Geometry: final body of the model. Coordinates: model frame, mm. Coordinates: 2 decimals unless noted, no trailing zeros. Write each loop counter-clockwise with the first axis right and the second up, starting at its lowest first coordinate (ties: lowest second). Pieces come first, ordered by that corner, then holes.
from build123d import *

# Parameters (mm, degrees)
F0_R     = 4
F0_R_2   = 1.5
F0_R_3   = 10
F1_DEPTH = 4


with BuildPart() as f1:
    # F0 (on Top) → F1 (new body)
    with BuildSketch(Plane.XY):
        with BuildLine():
            ThreePointArc((-44.266541, 56.889609), (-48.97612, 62.516223), (-51.339514, 69.462681))
            ThreePointArc((-51.339514, 69.462681), (-78.488853, 78.488853), (-69.462681, 51.339514))
            ThreePointArc((-69.462681, 51.339514), (-62.516223, 48.97612), (-56.889609, 44.266541))
            Line((-56.889609, 44.266541), (-33.507649, 15.901956))
            ThreePointArc((-33.507649, 15.901956), (-27.798264, 0), (-33.507649, -15.901956))
            Line((-33.507649, -15.901956), (-56.889609, -44.266541))
            ThreePointArc((-56.889609, -44.266541), (-62.516223, -48.97612), (-69.462681, -51.339514))
            ThreePointArc((-69.462681, -51.339514), (-78.488853, -78.488853), (-51.339514, -69.462681))
            ThreePointArc((-51.339514, -69.462681), (-48.97612, -62.516223), (-44.266541, -56.889609))
            Line((-44.266541, -56.889609), (-12.721564, -30.885937))
            ThreePointArc((-12.721564, -30.885937), (0, -26.318429), (12.721564, -30.885937))
            Line((12.721564, -30.885937), (44.266541, -56.889609))
            ThreePointArc((44.266541, -56.889609), (48.97612, -62.516223), (51.339514, -69.462681))
            ThreePointArc((51.339514, -69.462681), (78.488853, -78.488853), (69.462681, -51.339514))
            ThreePointArc((69.462681, -51.339514), (62.516223, -48.97612), (56.889609, -44.266541))
            Line((56.889609, -44.266541), (33.507649, -15.901956))
            ThreePointArc((33.507649, -15.901956), (27.798264, 0), (33.507649, 15.901956))
            Line((33.507649, 15.901956), (56.889609, 44.266541))
            ThreePointArc((56.889609, 44.266541), (62.516223, 48.97612), (69.462681, 51.339514))
            ThreePointArc((69.462681, 51.339514), (78.488853, 78.488853), (51.339514, 69.462681))
            ThreePointArc((51.339514, 69.462681), (48.97612, 62.516223), (44.266541, 56.889609))
            Line((44.266541, 56.889609), (12.721564, 30.885937))
            ThreePointArc((12.721564, 30.885937), (0, 26.318429), (-12.721564, 30.885937))
            Line((-12.721564, 30.885937), (-44.266541, 56.889609))
        make_face()
        with BuildLine():
            ThreePointArc((-72.831998, -70.710678), (-70.710678, -70.710678), (-70.710678, -72.831998))
            Line((-70.710678, -72.831998), (-72.831998, -74.953319))
            ThreePointArc((-72.831998, -74.953319), (-74.953319, -74.953319), (-74.953319, -72.831998))
            Line((-74.953319, -72.831998), (-72.831998, -70.710678))
        make_face(mode=Mode.SUBTRACT)
        with Locations((-67.175144, -67.175144)):
            Circle(F0_R, mode=Mode.SUBTRACT)
        with BuildLine():
            Line((-61.51829, -74.953319), (-63.63961, -72.831998))
            ThreePointArc((-63.63961, -72.831998), (-63.63961, -70.710678), (-61.51829, -70.710678))
            Line((-61.51829, -70.710678), (-59.39697, -72.831998))
            ThreePointArc((-59.39697, -72.831998), (-59.39697, -74.953319), (-61.51829, -74.953319))
        make_face(mode=Mode.SUBTRACT)
        with BuildLine():
            Line((-72.831998, -59.39697), (-70.710678, -61.51829))
            ThreePointArc((-70.710678, -61.51829), (-70.710678, -63.63961), (-72.831998, -63.63961))
            Line((-72.831998, -63.63961), (-74.953319, -61.51829))
            ThreePointArc((-74.953319, -61.51829), (-74.953319, -59.39697), (-72.831998, -59.39697))
        make_face(mode=Mode.SUBTRACT)
        with BuildLine():
            Line((-59.39697, -61.51829), (-61.51829, -63.63961))
            ThreePointArc((-61.51829, -63.63961), (-63.63961, -63.63961), (-63.63961, -61.51829))
            Line((-63.63961, -61.51829), (-61.51829, -59.39697))
            ThreePointArc((-61.51829, -59.39697), (-59.39697, -59.39697), (-59.39697, -61.51829))
        make_face(mode=Mode.SUBTRACT)
        with Locations((-15.25, -23)):
            Circle(F0_R_2, mode=Mode.SUBTRACT)
        with BuildLine():
            Line((-23, -9.5), (-23, 9.5))
            ThreePointArc((-23, 9.5), (-21.5, 11), (-20, 9.5))
            Line((-20, 9.5), (-20, -9.5))
            ThreePointArc((-20, -9.5), (-21.5, -11), (-23, -9.5))
        make_face(mode=Mode.SUBTRACT)
        with Locations((-15.25, -15.25)):
            Circle(F0_R_2, mode=Mode.SUBTRACT)
        with BuildLine():
            Line((59.39697, -72.831998), (61.51829, -70.710678))
            ThreePointArc((61.51829, -70.710678), (63.63961, -70.710678), (63.63961, -72.831998))
            Line((63.63961, -72.831998), (61.51829, -74.953319))
            ThreePointArc((61.51829, -74.953319), (59.39697, -74.953319), (59.39697, -72.831998))
        make_face(mode=Mode.SUBTRACT)
        with BuildLine():
            ThreePointArc((74.953319, -72.831998), (74.953319, -74.953319), (72.831998, -74.953319))
            Line((72.831998, -74.953319), (70.710678, -72.831998))
            ThreePointArc((70.710678, -72.831998), (70.710678, -70.710678), (72.831998, -70.710678))
            Line((72.831998, -70.710678), (74.953319, -72.831998))
        make_face(mode=Mode.SUBTRACT)
        with Locations((67.175144, -67.175144)):
            Circle(F0_R, mode=Mode.SUBTRACT)
        with BuildLine():
            ThreePointArc((63.63961, -61.51829), (63.63961, -63.63961), (61.51829, -63.63961))
            Line((61.51829, -63.63961), (59.39697, -61.51829))
            ThreePointArc((59.39697, -61.51829), (59.39697, -59.39697), (61.51829, -59.39697))
            Line((61.51829, -59.39697), (63.63961, -61.51829))
        make_face(mode=Mode.SUBTRACT)
        with BuildLine():
            ThreePointArc((72.831998, -63.63961), (70.710678, -63.63961), (70.710678, -61.51829))
            Line((70.710678, -61.51829), (72.831998, -59.39697))
            ThreePointArc((72.831998, -59.39697), (74.953319, -59.39697), (74.953319, -61.51829))
            Line((74.953319, -61.51829), (72.831998, -63.63961))
        make_face(mode=Mode.SUBTRACT)
        with Locations((15.25, -23)):
            Circle(F0_R_2, mode=Mode.SUBTRACT)
        with Locations((15.25, -15.25)):
            Circle(F0_R_2, mode=Mode.SUBTRACT)
        Circle(F0_R_3, mode=Mode.SUBTRACT)
        with BuildLine():
            ThreePointArc((20, 9.5), (21.5, 11), (23, 9.5))
            Line((23, 9.5), (23, -9.5))
            ThreePointArc((23, -9.5), (21.5, -11), (20, -9.5))
            Line((20, -9.5), (20, 9.5))
        make_face(mode=Mode.SUBTRACT)
        with Locations((-15.25, 15.25)):
            Circle(F0_R_2, mode=Mode.SUBTRACT)
        with Locations((-15.25, 23)):
            Circle(F0_R_2, mode=Mode.SUBTRACT)
        with BuildLine():
            ThreePointArc((-72.831998, 63.63961), (-70.710678, 63.63961), (-70.710678, 61.51829))
            Line((-70.710678, 61.51829), (-72.831998, 59.39697))
            ThreePointArc((-72.831998, 59.39697), (-74.953319, 59.39697), (-74.953319, 61.51829))
            Line((-74.953319, 61.51829), (-72.831998, 63.63961))
        make_face(mode=Mode.SUBTRACT)
        with BuildLine():
            ThreePointArc((-63.63961, 61.51829), (-63.63961, 63.63961), (-61.51829, 63.63961))
            Line((-61.51829, 63.63961), (-59.39697, 61.51829))
            ThreePointArc((-59.39697, 61.51829), (-59.39697, 59.39697), (-61.51829, 59.39697))
            Line((-61.51829, 59.39697), (-63.63961, 61.51829))
        make_face(mode=Mode.SUBTRACT)
        with Locations((-67.175144, 67.175144)):
            Circle(F0_R, mode=Mode.SUBTRACT)
        with BuildLine():
            ThreePointArc((-70.710678, 72.831998), (-70.710678, 70.710678), (-72.831998, 70.710678))
            Line((-72.831998, 70.710678), (-74.953319, 72.831998))
            ThreePointArc((-74.953319, 72.831998), (-74.953319, 74.953319), (-72.831998, 74.953319))
            Line((-72.831998, 74.953319), (-70.710678, 72.831998))
        make_face(mode=Mode.SUBTRACT)
        with BuildLine():
            ThreePointArc((-61.51829, 70.710678), (-63.63961, 70.710678), (-63.63961, 72.831998))
            Line((-63.63961, 72.831998), (-61.51829, 74.953319))
            ThreePointArc((-61.51829, 74.953319), (-59.39697, 74.953319), (-59.39697, 72.831998))
            Line((-59.39697, 72.831998), (-61.51829, 70.710678))
        make_face(mode=Mode.SUBTRACT)
        with Locations((15.25, 15.25)):
            Circle(F0_R_2, mode=Mode.SUBTRACT)
        with Locations((15.25, 23)):
            Circle(F0_R_2, mode=Mode.SUBTRACT)
        with BuildLine():
            Line((59.39697, 61.51829), (61.51829, 63.63961))
            ThreePointArc((61.51829, 63.63961), (63.63961, 63.63961), (63.63961, 61.51829))
            Line((63.63961, 61.51829), (61.51829, 59.39697))
            ThreePointArc((61.51829, 59.39697), (59.39697, 59.39697), (59.39697, 61.51829))
        make_face(mode=Mode.SUBTRACT)
        with BuildLine():
            Line((72.831998, 59.39697), (70.710678, 61.51829))
            ThreePointArc((70.710678, 61.51829), (70.710678, 63.63961), (72.831998, 63.63961))
            Line((72.831998, 63.63961), (74.953319, 61.51829))
            ThreePointArc((74.953319, 61.51829), (74.953319, 59.39697), (72.831998, 59.39697))
        make_face(mode=Mode.SUBTRACT)
        with BuildLine():
            Line((61.51829, 74.953319), (63.63961, 72.831998))
            ThreePointArc((63.63961, 72.831998), (63.63961, 70.710678), (61.51829, 70.710678))
            Line((61.51829, 70.710678), (59.39697, 72.831998))
            ThreePointArc((59.39697, 72.831998), (59.39697, 74.953319), (61.51829, 74.953319))
        make_face(mode=Mode.SUBTRACT)
        with Locations((67.175144, 67.175144)):
            Circle(F0_R, mode=Mode.SUBTRACT)
        with BuildLine():
            Line((74.953319, 72.831998), (72.831998, 70.710678))
            ThreePointArc((72.831998, 70.710678), (70.710678, 70.710678), (70.710678, 72.831998))
            Line((70.710678, 72.831998), (72.831998, 74.953319))
            ThreePointArc((72.831998, 74.953319), (74.953319, 74.953319), (74.953319, 72.831998))
        make_face(mode=Mode.SUBTRACT)
    extrude(amount=F1_DEPTH)


solid = f1.part
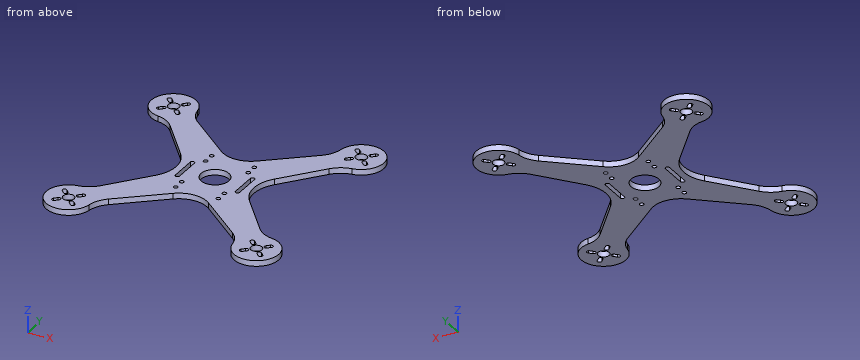
Item 1: Material intervals for probe 1 along X at (y, z) = (-69, 2.65); probe 2 along X at (y, z) = (-1, 3.35); probe 3 along X at (y, z) = (16, 0.2), sorted ascending.
Derived:
probe 1: x = -83.07 to -70.73, -63.62 to -51.27, 51.27 to 63.62, 70.73 to 83.07
probe 2: x = -27.82 to -23, -20 to -9.95, 9.95 to 20, 23 to 27.82
probe 3: x = -33.59 to -16.55, -13.95 to 13.95, 16.55 to 33.59
Item 2: Section D-D, the plane y = -49. Output: boundary loops of the cut face in (x, z).
Derived:
outline: (-62.56, 0) - (-34.7, 0) - (-34.7, 4) - (-62.56, 4) - close; (34.7, 0) - (62.56, 0) - (62.56, 4) - (34.7, 4) - close
Item 3: Section A-A, the plane y = 0. Output: boundary loops of the cut face in (x, z), plus the area to 3 significant figures.
Derived:
outline: (-27.8, 0) - (-23, 0) - (-23, 4) - (-27.8, 4) - close; (-20, 0) - (-10, 0) - (-10, 4) - (-20, 4) - close; (10, 0) - (20, 0) - (20, 4) - (10, 4) - close; (23, 0) - (27.8, 0) - (27.8, 4) - (23, 4) - close
area: 118 mm2
Item 4: Section C-C, the plane z = 3. State how many separate pieces and enclosed holes the cut face has, plus the area to 3 significant figures.
Derived:
separate pieces: 1
enclosed holes: 31
area: 9,350 mm2
Item 5: Pin query (flat end, axial travel): pin 1 (7 mm diameter, centred on x = -67.18, y = 67.18, fed in from -Z); pin 2 (1 mm diameter, centred on y = -49, z = 3.5, fed in from -X). Return the tip coordinate at first contact, or that it passes through.
Derived:
pin 1: passes through
pin 2: stops at x = -63.51
Item 6: Section B-B, the plane y = 33. Output: boundary loops of the cut face in (x, z).
Derived:
outline: (-47.6, 0) - (-15.29, 0) - (-15.29, 4) - (-47.6, 4) - close; (15.29, 0) - (47.6, 0) - (47.6, 4) - (15.29, 4) - close
